Can you work these out from the model? Positions are in its coordinate system, mm. A direction names the side the tool comes from. Round coordinates to 2 decimals unless told otherwise and drop trailing zeros. Write each loop counter-clockwise with the first axis right and the second up, starting at its lowest first coordinate (ties: lowest second). Pieces come first, ordered by that corner, then holes. Notation, with made-up numbers: M 58,-20 L 103,-20 A10 ccw 103,-4 Z; hole C 79.25,-24.5 d5. An arc over 180 degrees is marked long. Answer in a Markdown table with one row per item. Add a question column.
(1) If I drill on probe 1 along Z at (x, y) = (0, 50); probe 2 along Z at (x, y) = (0, 20); probe 3 along Z at (x, y) = (2.25, 54.5), over which ranges is the centre line in solid material (lowest first)?
(2) For faces 1 (the face through (0, 33, 5)), 2 (the face through (0, 48, -4)), 3 (the face through (1.5, 110, -0.7)), which set-ups out of +Z, -Z, +X, -X, +Y, -Y let a thin tool reach every point of the face, with its end or its side?
(3) Suppose I cut it at B-B, the plane z = 0. Write out the boundary of the cut face in (x, y), then the cut area to 3 significant figures.
(4) Suppose I cut it at C-C, the plane y = 15. Write out the boundary of the cut face in (x, z), then the cut area to 3 significant figures.
(5) Suppose I cut it at D-D, the plane x = 5.75. Write out the boundary of the cut face in (y, z), then the cut area to 3 significant figures.
(6) I'm going to push flat-ended pins straight in: pin 1 (3 mm diameter, centred on y = 23, z = 4.5, fed in from -X); pin 2 (4 mm diameter, centred on y = 12, z = 1.5, fed in from +X); pin 3 (1 mm diameter, centred on x = 0, z = 0.5, fed in from -Y); pin 4 (1.5 mm diameter, centred on x = -3.5, y = 54.5, fed in from +Z). Where does each tip first touch, or does it pass through?
(7) Suppose I cut it at A-A, the plane y = 51.5. Write out the boundary of the cut face in (x, z), then the cut area to 3 significant figures.
from build123d import *

# Parameters (mm, degrees)
F0_R     = 5
F3_DEPTH = 110
F5_DEPTH = 33


with BuildPart() as f2:
    # F1 (on Right) → F2 (revolve)
    with BuildSketch(Plane.YZ):
        Polygon((0, 5.5), (0, 4), (95, 4), (110, 1.5), (110, 5.5), (95, 5.5), align=None)
    revolve(axis=Axis((0, 47.5, 0), (0, 1, 0)))

    # F0 (on Front) → F3 (join)
    with BuildSketch(Plane.XZ):
        Polygon((4.4083893922, -6.0676274578), (7.1329238722, 2.3176274578), (0, 7.5), (-7.1329238722, 2.3176274578), (-4.4083893922, -6.0676274578), align=None)
        Circle(F0_R, mode=Mode.SUBTRACT)
    extrude(amount=-F3_DEPTH)

    # F4 (on face) → F5 (cut)
    with BuildSketch(Plane.XZ):
        with BuildLine():
            Line((-2.5, 5.68364368), (-2.5, 3.1224989992))
            ThreePointArc((-2.5, 3.1224989992), (-1.3247648854, 3.7742546282), (0, 4))
            Line((0, 4), (0, 7.5))
            Line((0, 7.5), (-2.5, 5.68364368))
        make_face()
        with BuildLine():
            ThreePointArc((0, 4), (1.3247648854, 3.7742546282), (2.5, 3.1224989992))
            Line((2.5, 3.1224989992), (2.5, 5.68364368))
            Line((2.5, 5.68364368), (0, 7.5))
            Line((0, 7.5), (0, 4))
        make_face()
    extrude(amount=-F5_DEPTH, mode=Mode.SUBTRACT)


solid = f2.part
Calculated:
| question | item | result |
|---|---|---|
| 1 | probe 1 | -6.07 to -4, 4 to 7.5 |
| 1 | probe 2 | -6.07 to -4 |
| 1 | probe 3 | -6.07 to -3.31, 3.31 to 5.87 |
| 2 | face 1 | +Z, -Y |
| 2 | face 2 | -Y |
| 2 | face 3 | +Z, -Z, +X, -X, +Y |
| 3 | outline | M -6.38,0 L -4,0 L -4,95 L -1.5,110 L -6.38,110 Z; M 1.5,110 L 4,95 L 4,0 L 6.38,0 L 6.38,110 Z |
| 3 | area | 561 mm² |
| 4 | outline | M -7.13,2.32 L -4.41,-6.07 L 4.41,-6.07 L 7.13,2.32 L 2.5,5.68 L 2.5,3.12 A4 cw long -2.5,3.12 L -2.5,5.68 Z |
| 4 | area | 69.1 mm² |
| 5 | outline | M 0,-1.94 L 110,-1.94 L 110,3.32 L 0,3.32 Z |
| 5 | area | 579 mm² |
| 6 | pin 1 | x = -6.19 |
| 6 | pin 2 | x = 7.13 |
| 6 | pin 3 | through |
| 6 | pin 4 | z = 5.5 |
| 7 | outline | M -7.13,2.32 L -4.41,-6.07 L 4.41,-6.07 L 7.13,2.32 L 0,7.5 Z; hole C 0,0 d8 |
| 7 | area | 83.5 mm² |
